Geometry check sheet. Reference: the model listing, model coordinates, mm. A direction names the side the tool comes from. Round coordinates to 2 decimals unless told otherwise and drop trailing zeros. Order: outer loops, then holes, each group sorted by start corner. A loop starts at its lowest first (then second) coordinate and runs counter-clockwise, first axis right, second up. Notation, with made-up numbers: (11.25, 52.5) - (52.25, 52.5) arc R29 ccw to (52.25, 74.5) - close; hole circle Ø10 at (-2, 0). An arc over 180 degrees is marked (long way). Write each question's results on one line, items separated by ' | '.
```python
from build123d import *

# Parameters (mm, degrees)
F1_DEPTH = 2.5
F2_R     = 5


with BuildPart() as f1:
    # F0 (on Front) → F1 (new body)
    with BuildSketch(Plane.XZ):
        with BuildLine():
            ThreePointArc((17.224815, 8.702017), (18.191599, 9.333046), (18.003069, 10.472047))
            ThreePointArc((18.003069, 10.472047), (-35.240268, 33.882295), (-88.483606, 10.472047))
            ThreePointArc((-88.483606, 10.472047), (-88.672136, 9.333046), (-87.705352, 8.702017))
            Line((-87.705352, 8.702017), (-79.325233, 8.702017))
            ThreePointArc((-79.325233, 8.702017), (-68.207651, 16.241039), (-59.327855, 6.162017))
            ThreePointArc((-59.327855, 6.162017), (-68.207651, -3.917004), (-79.325233, 3.622017))
            Line((-79.325233, 3.622017), (-87.705352, 3.622017))
            ThreePointArc((-87.705352, 3.622017), (-88.672136, 2.990989), (-88.483606, 1.851987))
            ThreePointArc((-88.483606, 1.851987), (-35.240268, -21.558261), (18.003069, 1.851987))
            ThreePointArc((18.003069, 1.851987), (18.191599, 2.990989), (17.224815, 3.622017))
            Line((17.224815, 3.622017), (9.087631, 3.622017))
            ThreePointArc((9.087631, 3.622017), (-10.909747, 6.162017), (9.087631, 8.702017))
            Line((9.087631, 8.702017), (17.224815, 8.702017))
        make_face()
    extrude(amount=F1_DEPTH)

    # F2
    f2_edges = [f1.edges().sort_by_distance(p)[0] for p in [
        (-79.325233, -1.25, 3.622017),
        (-79.325233, -1.25, 8.702017),
        (9.087631, -1.25, 8.702017),
        (9.087631, -1.25, 3.622017),
    ]]
    fillet(f2_edges, radius=F2_R)


solid = f1.part
```
(1) Section check B-B (y = -1.6). Record the cut outline in (x, z), then the cut area to 3 significant figures.
Answers follow:
outline: (-88.48, 1.85) arc R72.25 ccw to (18, 1.85) arc R1.06 ccw to (17.22, 3.62) - (12.4, 3.62) arc R5 ccw to (8.06, 1.11) arc R10.16 cw (long way) to (8.06, 11.22) arc R5 ccw to (12.4, 8.7) - (17.22, 8.7) arc R1.06 ccw to (18, 10.47) arc R72.25 ccw to (-88.48, 10.47) arc R1.06 ccw to (-87.71, 8.7) - (-82.64, 8.7) arc R5 ccw to (-78.3, 11.22) arc R10.16 cw (long way) to (-78.3, 1.11) arc R5 ccw to (-82.64, 3.62) - (-87.71, 3.62) arc R1.06 ccw to start | area: 3,620 mm²
(2) Section check D-D (z = -18). Record the cut outline in (x, y), then the cut area to 3 significant figures.
Answers follow:
outline: (-57.64, -2.5) - (-12.85, -2.5) - (-12.85, 0) - (-57.64, 0) - close | area: 112 mm²
(3) Depth check by flat-ended pin: pin 1 Ø0.8 at (x, y) = (16, -1) entering from +Z; pin 2 Ø1 at (y, z) = (-2, -2.5) entering from +X; pin 3 Ø1.2 at (x, y) = (16, -1.5) entering from -Z. Enter the tip coordinate at first touch or a pass-through.
Answers follow:
pin 1: z = 12.97 | pin 2: x = 14.19 | pin 3: z = -0.84
(4) Section check A-A (x = -61.5). Record the cut outline in (y, z), then the cut area to 3 significant figures.
Answers follow:
outline: (-2.5, -16.62) - (0, -16.62) - (0, -0.12) - (-2.5, -0.12) - close; (-2.5, 12.44) - (0, 12.44) - (0, 28.94) - (-2.5, 28.94) - close | area: 82.5 mm²
(5) Material ranges on line 1 (X direction, y = -0.6, z = 1.5); line 2 (X direction, y = -1.8, z = 13.5); line 3 (Z direction, x = 5, y = -0.3), recorded low to high.
Answers follow:
line 1: -88.16 to -78.55, -60.46 to -9.78, 8.31 to 17.68 | line 2: -85.54 to -76.51, -62.46 to -7.78, 6.28 to 15.06 | line 3: -9.32 to -2.21, 14.54 to 21.64
(6) Draft check along Y on faces 1 (the face through (-36, -2.5, 7)), 2 (the face through (-80.1, -1.27, 2.93)), 3 (the face through (-36, 0, 7)). Enter one of: released by +Y, released by -Y, zero draft, split by the parting line, or undercut.
Answers follow:
face 1: released by -Y | face 2: zero draft | face 3: released by +Y
(7) Section check C-C (x = -8). Record the cut outline in (y, z), then the cut area to 3 significant figures.
Answers follow:
outline: (-2.5, -16.23) - (0, -16.23) - (0, -0.96) - (-2.5, -0.96) - close; (-2.5, 13.28) - (0, 13.28) - (0, 28.55) - (-2.5, 28.55) - close | area: 76.4 mm²
(8) Access from +Z, -Z, +X, -X, +Y, -Y to the whole of each face (thin tool, end or side, straight path). Record for faces 4 (the face through (-85, -1, 3.622)), 5 (the face through (9.864, -1.268, 9.394)), 6 (the face through (15, -1, 3.622)).
Answers follow:
face 4: -X, +Y, -Y | face 5: +Y, -Y | face 6: +X, +Y, -Y
